```python
from build123d import *

# Parameters (mm, degrees)
SKETCH1_W           = 6
SKETCH1_H           = 10
SKETCH1_R           = 1
BOSS_EXTRUDE1_DEPTH = 2
BOSS_EXTRUDE2_DEPTH = 2
SKETCH3_W           = 8
SKETCH3_H           = 20
BOSS_EXTRUDE3_DEPTH = 1
SKETCH4_R           = 1
CUT_EXTRUDE1_DEPTH  = 5
LPATTERN1_COUNT     = 3
LPATTERN1_PITCH     = 6
CHAMFER1_SIZE       = 5
FILLET1_R           = 2


with BuildPart() as part:
    # Sketch1 → Boss-Extrude1 (new body)
    with BuildSketch(Plane.XY):
        Rectangle(SKETCH1_W, SKETCH1_H)
        with Locations((0, 1.75)):
            Circle(SKETCH1_R, mode=Mode.SUBTRACT)
        with Locations((0, -1.75)):
            Circle(SKETCH1_R, mode=Mode.SUBTRACT)
    extrude(amount=BOSS_EXTRUDE1_DEPTH)

    # Sketch2 → Boss-Extrude2 (add)
    with BuildSketch(Plane.XY.offset(2)):
        Polygon((-14, -10), (-14, 10), (-6, 10), (-6, 5), (-3, 5), (-3, -5), (-6, -5), (-6, -10), align=None)
    extrude(amount=-BOSS_EXTRUDE2_DEPTH)

    # Sketch3 → Boss-Extrude3 (add)
    with BuildSketch(Plane(origin=(0, 0, 0), x_dir=(-1, 0, 0), z_dir=(0, 0, -1))):
        with Locations((10, 0)):
            Rectangle(SKETCH3_W, SKETCH3_H)
    extrude(amount=BOSS_EXTRUDE3_DEPTH)

    # Sketch4 → Cut-Extrude1 (cut)
    with BuildSketch(Plane.XY.offset(2)):
        with Locations((-8.5, -7.5)):
            Circle(SKETCH4_R)
        with Locations((-11.5, -4.5)):
            Circle(SKETCH4_R)
    cut_extrude1 = extrude(amount=-CUT_EXTRUDE1_DEPTH, mode=Mode.SUBTRACT)

    # LPattern1: Cut-Extrude1 ×3
    with Locations(*[(0, i * LPATTERN1_PITCH, 0) for i in range(1, LPATTERN1_COUNT)]):
        add(cut_extrude1, mode=Mode.SUBTRACT)

    # Chamfer1
    chamfer1_edges = [part.edges().sort_by_distance(p)[0] for p in [
        (-6, 5, 1),
        (-6, -5, 1),
    ]]
    chamfer(chamfer1_edges, length=CHAMFER1_SIZE - 0.0001)  # a hair under: the kernel refuses the full size

    # Fillet1
    fillet1_edges = [part.edges().sort_by_distance(p)[0] for p in [
        (-14, -10, 0.5),
        (-14, 10, 0.5),
        (3, -5, 1),
        (3, 5, 1),
    ]]
    fillet(fillet1_edges, radius=FILLET1_R)


solid = part.part
```
Can you work these out from the model? Positions are in its coordinate system, mm. A direction names the side the tool comes from. Coordinates: 2 decimals unless noted, no trailing zeros. Loops run counter-clockwise (first coordinate to the right, second up) from the corner with the lowest first, then second, coordinate; pieces in that order, holes last. Notation, with made-up numbers: (-21, 5) -> (1, 5) arc R24 cw to (1, 32) -> close; hole circle Ø11 at (58.25, 67). An arc over 180 degrees is marked (long way). Answer as a JSON object with one key per item and string values.
1) If I drill on line 1 (Y direction, x = -8.5, z = 0.6); line 2 (Y direction, x = -11.5, z = 0.2); line 3 (Y direction, x = 0.25, z = 0.1), over which ranges is the centre line in solid material (lowest first)?
Results:
{"line 1": "y = -10 to -8.5, -6.5 to -2.5, -0.5 to 3.5, 5.5 to 10", "line 2": "y = -10 to -5.5, -3.5 to 0.5, 2.5 to 6.5, 8.5 to 10", "line 3": "y = -5 to -2.72, -0.78 to 0.78, 2.72 to 5"}
2) Thinking about a two-plate mould opening in Y: for faces 1 (the face through (-9.3, -2.1, 0.5)), 2 (the face through (-13.4, 9.43, 0.52)), 3 (the face through (0, -5, 1)), which applies, pulls with the +Y half, pulls with the -Y half, needs draft (parallel to the pull), parting line crosses it, or undercut?
Results:
{"face 1": "undercut", "face 2": "pulls with the +Y half", "face 3": "pulls with the -Y half"}
3) For faces 4 (the face through (-6, 0, -0.4)), 5 (the face through (-13.43, -9.4, 0.48)), 6 (the face through (0, 5, 1)), which set-ups out of +Z, -Z, +X, -X, +Y, -Y let a thin tool reach every point of the face, with its end or its side?
Results:
{"face 4": "-Z, +X, +Y, -Y", "face 5": "+Z, -Z, -X, -Y", "face 6": "+Z, -Z, +X, +Y"}
4) Imagine slicing it at A-A (x = -8.5). Please give me the cut outline in (y, z), then the cut area to 3 significant figures.
Results:
{"outline": "(-10, -1) -> (-8.5, -1) -> (-8.5, 2) -> (-10, 2) -> close; (-6.5, -1) -> (-2.5, -1) -> (-2.5, 2) -> (-6.5, 2) -> close; (-0.5, -1) -> (3.5, -1) -> (3.5, 2) -> (-0.5, 2) -> close; (5.5, -1) -> (10, -1) -> (10, 2) -> (5.5, 2) -> close", "area": "42.0 mm^2"}
5) For P1, Ø2.5, axis at x = -2, y = -3, coming from the -Z side; P2, Ø1, axis at x = 0, z = 0.5, coming from the +Y side; P3, Ø1.5, axis at y = 4.5, z = 0, coming from the +X side, each with a flat end and sliding along its axis, tell me the tip position at first contact or that it passes through.
Results:
{"P1": "stops at z = 0", "P2": "stops at y = 5", "P3": "stops at x = 2.85"}
6) Imagine slicing it at C-C (y = 1.75). Please give me the cut outline in (x, z), then the cut area to 3 significant figures.
Results:
{"outline": "(-14, -1) -> (-12.47, -1) -> (-12.47, 2) -> (-14, 2) -> close; (-10.53, -1) -> (-6, -1) -> (-6, 0) -> (-1, 0) -> (-1, 2) -> (-10.53, 2) -> close; (1, 0) -> (3, 0) -> (3, 2) -> (1, 2) -> close", "area": "32.2 mm^2"}
7) Imagine slicing it at D-D (x = 0). Please give me the cut outline in (y, z).
Results:
{"outline": "(-5, 0) -> (-2.75, 0) -> (-2.75, 2) -> (-5, 2) -> close; (-0.75, 0) -> (0.75, 0) -> (0.75, 2) -> (-0.75, 2) -> close; (2.75, 0) -> (5, 0) -> (5, 2) -> (2.75, 2) -> close"}
8) Imagine slicing it at B-B (z = 0.95). Count the separate pieces of the cut face and the enclosed holes in it, then the cut area to 3 significant figures.
Results:
{"separate pieces": "1", "enclosed holes": "8", "area": "246 mm^2"}
